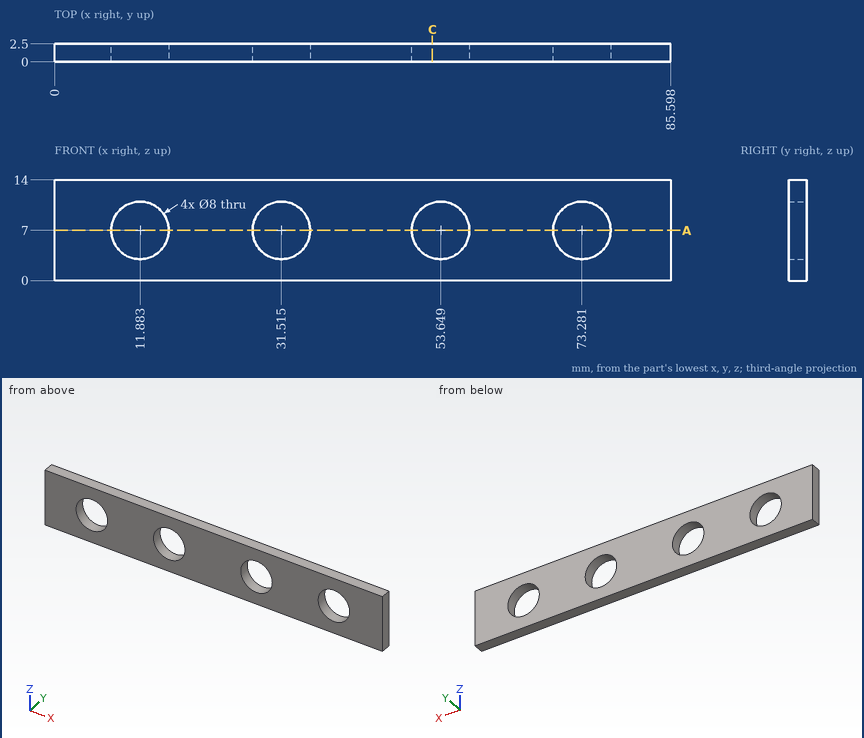
Geometry check sheet. Reference: drawing and pictorial views, mm from the part's lowest x, y, z. Give positions to 0.01 mm unless a question says otherwise; leave off trailing zeros. Write each loop counter-clockwise with the first axis right and the second up, starting at its lowest first coordinate (ties: lowest second). Pieces come first, ordered by that corner, then holes. Notation, with made-up numbers: M -33.5,-16 L -1.5,-16 A23 cw -1.5,9 Z; hole C 25.5,9.25 d7. An arc over 180 degrees is marked long. Put each result on its own line as item: value. Start each with the question number.
1. Section check C-C (x = 52.5). Record the cut outline in (y, z).
2. Section check A-A (z = 7). Give the number of separate pieces and of enclosed holes in the cut face, and give its area (3 significant figures).
3. Scan lines: line 1 along Z through (x, y) = (53.5, 0.75); line 2 along Z through (x, y) = (52, 0.15) (1 decimal); line 3 along X through (y, z) = (1.85, 5.25) (1 decimal). Record each from-to range of solid material in increasing order. Write a range as [from, to].
Answer list:
1. outline: M 0,0 L 2.5,0 L 2.5,3.17 L 0,3.17 Z; M 0,10.83 L 2.5,10.83 L 2.5,14 L 0,14 Z
2. separate pieces: 5
2. enclosed holes: 0
2. area: 134 mm2
3. line 1: [0, 3], [11, 14]
3. line 2: [0, 3.4], [10.6, 14]
3. line 3: [0, 8.3], [15.5, 27.9], [35.1, 50.1], [57.2, 69.7], [76.9, 85.6]
